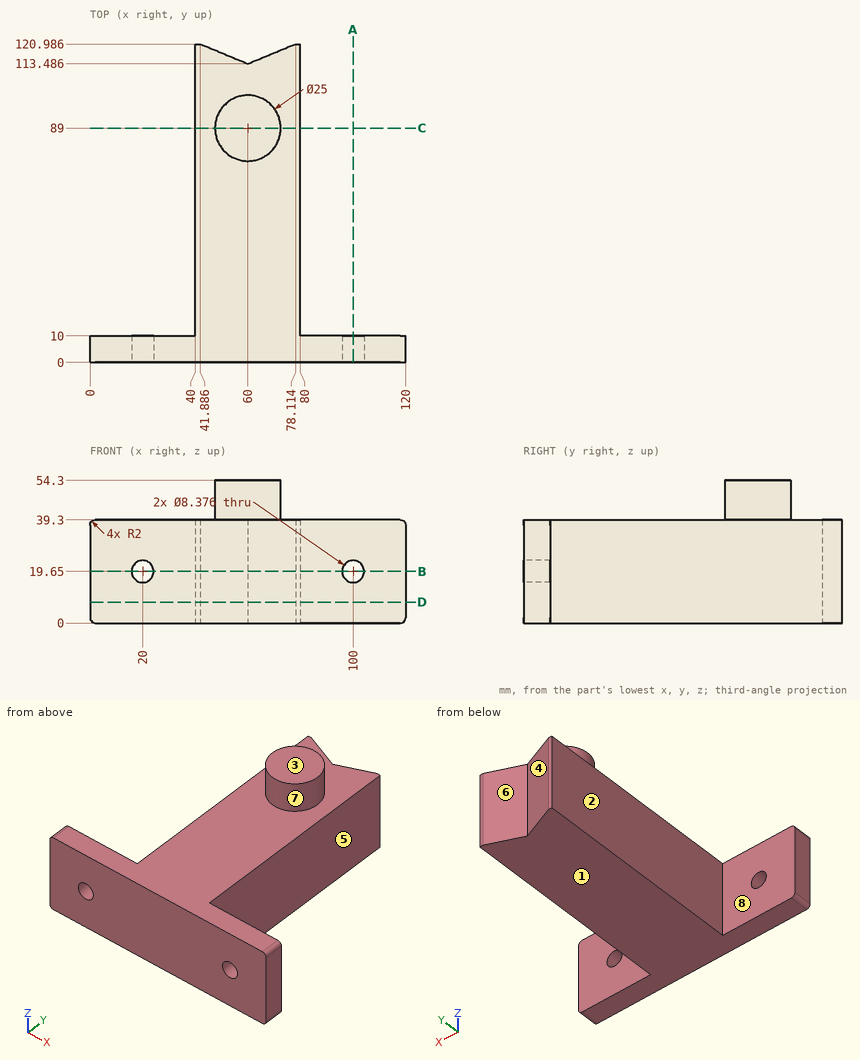
Job drawing, mm, ordinate dimensions from the low corner. One solid piece. A direction names the side the tool comes from. Round coordinates to 2 decimals unless told otherwise and drop trailing zeros. Write each loop counter-clockwise with the first axis right and the second up, starting at its lowest first coordinate (ties: lowest second). Pieces come first, ordered by that corner, then holes. Notation, with made-up numbers: M 11,72 L 63,72 A24 cw 63,103 Z; hole C -2.5,-14 d6. An arc over 180 degrees is marked long. Return JSON: item names as keys, results as strings. Group by question number.
(1) Saw through at D-D on z = 8. Write the cut outline in (x, y) (1 decimal).
(2) Pin check, flat tips, straight feed: pin 1 Ø12 at (x, z) = (105, 21.5) entering from +Y; pin 2 Ø8 at (y, z) = (31.5, 12.5) entering from -X; pin 3 Ø2 at (x, z) = (56, 9) entering from +Y; pin 4 Ø5 at (x, z) = (14.5, 36) entering from -Y. Stop position of each tip, or through.
(3) Saw through at C-C on y = 89. Write the cut outline in (x, z).
(4) Saw through at A-A on x = 100. Write the cut outline in (y, z).
(5) Drill centre lines: probe 1 along X at (y, z) = (4, 19.65); probe 2 along Z at (x, y) = (20, 5.25); probe 3 along Y at (x, z) = (35, 37.5). Where is each one in solid material? Low to high.
(6) Saw through at B-B on z = 19.65. Write the cut outline in (x, y) (1 decimal).
(7) Which spindle directions (+Z, -Z, +X, -X, +Y, -Y) get a long thin tool onto all of the face, cutting with end or side? Do the marked faces 1, 2, 3, 4 and 5. Say none if no direction does.
(8) Two-plate mould, pull along X, no slides. Class the marked faces 6, 7 and 8: +X half, -X half, draft (parallel to the pull), parting line (faces both ways), or undercut.
Returned:
{
 "1": {"outline": "M 0,0 L 120,0 L 120,10 L 80,10 L 80,121 L 78.1,121 L 60,113.5 L 41.9,121 L 40,121 L 40,10 L 0,10 Z"},
 "2": {"pin 1": "y = 10", "pin 2": "x = 40", "pin 3": "y = 115.56", "pin 4": "y = 0"},
 "3": {"outline": "M 40,0 L 80,0 L 80,39.3 L 72.5,39.3 L 72.5,54.3 L 47.5,54.3 L 47.5,39.3 L 40,39.3 Z"},
 "4": {"outline": "M 0,0 L 10,0 L 10,15.46 L 0,15.46 Z; M 0,23.84 L 10,23.84 L 10,39.3 L 0,39.3 Z"},
 "5": {"probe 1": "0 to 15.81, 24.19 to 95.81, 104.19 to 120", "probe 2": "0 to 15.46, 23.84 to 39.3", "probe 3": "0 to 10"},
 "6": {"outline": "M 0,0 L 15.8,0 L 15.8,10 L 0,10 Z; M 24.2,0 L 95.8,0 L 95.8,10 L 80,10 L 80,121 L 78.1,121 L 60,113.5 L 41.9,121 L 40,121 L 40,10 L 24.2,10 Z; M 104.2,0 L 120,0 L 120,10 L 104.2,10 Z"},
 "7": {"face 1": "-Z, +X, -X, +Y, -Y", "face 2": "+Z, -Z, -X, +Y", "face 3": "+Z, +X, -X, +Y, -Y", "face 4": "+Z, -Z, +Y", "face 5": "+Z, -Z, +X, +Y"},
 "8": {"face 6": "undercut", "face 7": "parting line", "face 8": "draft"}
}
